Here's how the part is built. I have some questions about the finished solid (model axes, mm). A direction names the side the tool comes from. Give positions to 0.01 mm unless a question says otherwise; leave off trailing zeros. Loops run counter-clockwise (first coordinate to the right, second up) from the corner with the lowest first, then second, coordinate; pieces in that order, holes last.
Q1. Suppose I cut it at C-C (z = -13). List the corners of the cut face in (x, y) for me, and give its area (3 significant figures).
Q2. For faces 1 (the face through (13.7, 1, -5)), 2 (the face through (7.8, 0.5, -2.6)), 3 (the face through (28.49, 1, -42)), which set-ups out of +Z, -Z, +X, -X, +Y, -Y let a thin tool reach every point of the face, with its end or its side?
Q3. Thinking about a two-plate mould opening in Z: for faces 4 (the face through (23.38, 1.514, -69.117)), 5 (the face through (14, 0, -39)), 6 (the face through (14, 1, -75.5)), 7 (the face through (21, 1, -9.5)), which applies, pulls with the +Z half, pulls with the -Z half, needs draft (parallel to the pull), parting line crosses it, or undercut?
Q4. Suppose I cut it at D-D (x = 7.5). List the corners of the cut face in (y, z) for me.
Q5. I need wall thicknesses on probe 1 along Z at (x, y) = (7.5, 0.2); probe 2 along Z at (x, y) = (21.31, 1.45); probe 3 along X at (y, z) = (1.4, -65.5). Which ranges of each line are inside material? Lowest first, please.
Q6. I'm going to push flat-ended pins straight in: P1, Ø4.5, axis at x = 21.31, z = -13, coming from the +Y side; P2, Ø1.2, axis at x = 18, y = 1, coming from the +Z side; P3, Ø0.8, axis at y = 1, z = -7, coming from the +X side. Where does each tip first touch, or does it pass through?
Q7. Suppose I cut it at A-A (y = 1.55). List the corners of the cut face in (x, z) for me.
Q8. Suppose I cut it at B-B (x = 21.88). List the corners of the cut face in (y, z) for me, and give its area (3 significant figures).
```python
from build123d import *

# Parameters (mm, degrees)
BOSS_EXTRUDE1_DEPTH                         = 2.5
CBORE_FOR_M3_CHEESE_HEAD_SCREW1_D           = 3.4
CBORE_FOR_M3_CHEESE_HEAD_SCREW1_CBORE_D     = 6.5
CBORE_FOR_M3_CHEESE_HEAD_SCREW1_CBORE_DEPTH = 2
CUT_EXTRUDE1_DEPTH                          = 10
SKETCH6_W                                   = 14.59
SKETCH6_H                                   = 0.5
CUT_EXTRUDE2_DEPTH                          = 10
CUT_EXTRUDE3_DEPTH                          = 10
SKETCH8_W                                   = 0.2
SKETCH8_H                                   = 9.000000433
CUT_EXTRUDE4_DEPTH                          = 10


with BuildPart() as part:
    # Sketch1 → Boss-Extrude1 (new body)
    with BuildSketch(Plane(origin=(0, 0, 0), x_dir=(1, 0, 0), z_dir=(0, 1, 0))):
        Polygon((0, 0), (13.9, 0), (13.9, 9), (28.49, 9), (28.49, 76), (-0.1, 76), align=None)
    extrude(amount=BOSS_EXTRUDE1_DEPTH)

    # CBORE for M3 Cheese Head Screw1 (through all)
    with Locations(Plane(origin=(0, 2.5, 0), x_dir=(1, 0, 0), z_dir=(0, 1, 0))):
        with Locations((6.835263153, 72.000003463), (21.88, 72.000003463), (21.31, 13), (6.444736847, 3.999996537)):
            CounterBoreHole(CBORE_FOR_M3_CHEESE_HEAD_SCREW1_D / 2, CBORE_FOR_M3_CHEESE_HEAD_SCREW1_CBORE_D / 2, CBORE_FOR_M3_CHEESE_HEAD_SCREW1_CBORE_DEPTH)

    # Sketch5 → Cut-Extrude1 (cut)
    with BuildSketch(Plane(origin=(0, 2.5, 0), x_dir=(1, 0, 0), z_dir=(0, 1, 0))):
        Polygon((-0.1, 76), (-0.099342106, 75.500000433), (28.49, 75.500000433), (28.49, 76), align=None)
    extrude(amount=-CUT_EXTRUDE1_DEPTH, mode=Mode.SUBTRACT)

    # Sketch6 → Cut-Extrude2 (cut)
    with BuildSketch(Plane(origin=(0, 2.5, 0), x_dir=(1, 0, 0), z_dir=(0, 1, 0))):
        with Locations((21.195, 9.25)):
            Rectangle(SKETCH6_W, SKETCH6_H)
    extrude(amount=-CUT_EXTRUDE2_DEPTH, mode=Mode.SUBTRACT)

    # Sketch7 → Cut-Extrude3 (cut)
    with BuildSketch(Plane(origin=(0, 2.5, 0), x_dir=(1, 0, 0), z_dir=(0, 1, 0))):
        Polygon((13.9, 0), (13.9, 0.499999567), (-0.000657894, 0.499999567), (0, 0), align=None)
    extrude(amount=-CUT_EXTRUDE3_DEPTH, mode=Mode.SUBTRACT)

    # Sketch8 → Cut-Extrude4 (cut)
    with BuildSketch(Plane(origin=(0, 2.5, 0), x_dir=(1, 0, 0), z_dir=(0, 1, 0))):
        with Locations((13.8, 4.999999783)):
            Rectangle(SKETCH8_W, SKETCH8_H)
    extrude(amount=-CUT_EXTRUDE4_DEPTH, mode=Mode.SUBTRACT)


solid = part.part
```
Solutions:
1. outline: (-0.02, 0) - (19.61, 0) - (19.61, 0.5) - (18.06, 0.5) - (18.06, 2.5) - (-0.02, 2.5) - close; (23.01, 0) - (28.49, 0) - (28.49, 2.5) - (24.56, 2.5) - (24.56, 0.5) - (23.01, 0.5) - close
1. area: 56.6 mm2
2. face 1: +Z, +X, +Y, -Y
2. face 2: +Y
2. face 3: +Z, -Z, +X, +Y, -Y
3. face 4: undercut
3. face 5: needs draft
3. face 6: pulls with the -Z half
3. face 7: pulls with the +Z half
4. outline: (0, -75.5) - (2.5, -75.5) - (2.5, -75.18) - (0.5, -75.18) - (0.5, -73.56) - (0, -73.56) - close; (0, -70.44) - (0.5, -70.44) - (0.5, -68.82) - (2.5, -68.82) - (2.5, -7.07) - (0.5, -7.07) - (0.5, -5.33) - (0, -5.33) - close; (0, -2.67) - (0.5, -2.67) - (0.5, -0.93) - (2.5, -0.93) - (2.5, -0.5) - (0, -0.5) - close
5. probe 1: z = -75.5 to -73.56, -70.44 to -5.33, -2.67 to -0.5
5. probe 2: z = -75.5 to -75.2, -68.8 to -16.25, -9.75 to -9.5
5. probe 3: x = -0.09 to 28.49
6. P1: stops at y = 0.5
6. P2: stops at z = -9.5
6. P3: stops at x = 13.7
7. outline: (-0.1, -75.5) - (28.49, -75.5) - (28.49, -9.5) - (13.7, -9.5) - (13.7, -0.5) - (0, -0.5) - close; hole circle Ø6.5 at (6.44, -4); hole circle Ø6.5 at (6.84, -72); hole circle Ø6.5 at (21.31, -13); hole circle Ø6.5 at (21.88, -72)
8. outline: (0, -75.5) - (2.5, -75.5) - (2.5, -75.25) - (0.5, -75.25) - (0.5, -73.7) - (0, -73.7) - close; (0, -70.3) - (0.5, -70.3) - (0.5, -68.75) - (2.5, -68.75) - (2.5, -16.2) - (0.5, -16.2) - (0.5, -14.6) - (0, -14.6) - close; (0, -11.4) - (0.5, -11.4) - (0.5, -9.8) - (2.5, -9.8) - (2.5, -9.5) - (0, -9.5) - close
8. area: 136 mm2
